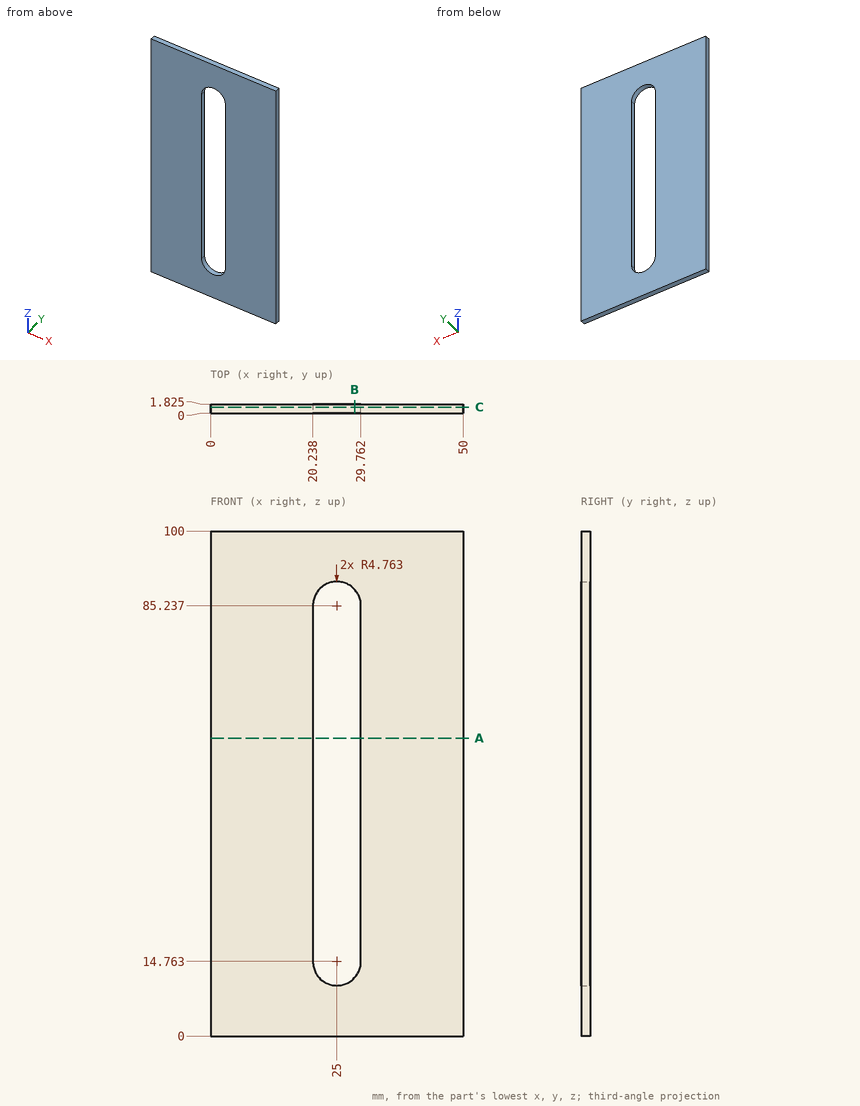
The figure shows three views and two pictorial views of one solid part (mm, origin at its lowest corner). Answer the questions. Round coordinates to 2 decimals unless told otherwise and drop trailing zeros. Write each loop counter-clockwise with the first axis right and the second up, starting at its lowest first coordinate (ties: lowest second). Pieces come first, ordered by that corner, then holes. Notation, with made-up numbers: (34, 48) - (46, 48) arc R9 cw to (46, 55) - close; hole circle Ø10 at (46.5, 42.5). An arc over 180 degrees is marked (long way). Answer in a Markdown table with one row per item. Add a question column.
1. A cutting plane is placed at B-B, the plane x = 28.5. Determine the outline of the cut face in (y, z) (1 decimal).
2. Find the intervals of material crossed by line 1 along X through (y, z) = (1.1, 36); line 2 along X through (y, z) = (0.55, 86.5); line 3 along Z through (x, y) = (28, 0.75) (1 decimal), in increasing order. Write a range as from..to.
3. A cutting plane is placed at A-A, the plane z = 59. Determine the outline of the cut face in (x, y) (1 decimal).
4. A cutting plane is placed at C-C, the plane y = 1.2. Determine the outline of the cut face in (x, z) (1 decimal), and give its area (3 significant figures).
Worked out:
| question | item | result |
|---|---|---|
| 1 | outline | (0, 0) - (1.8, 0) - (1.8, 11.5) - (0, 11.5) - close; (0, 88.5) - (1.8, 88.5) - (1.8, 100) - (0, 100) - close |
| 2 | line 1 | 0..20.24, 29.76..50 |
| 2 | line 2 | 0..20.41, 29.59..50 |
| 2 | line 3 | 0..11.1, 88.9..100 |
| 3 | outline | (0, 0) - (20.2, 0) - (20.2, 1.8) - (0, 1.8) - close; (29.8, 0) - (50, 0) - (50, 1.8) - (29.8, 1.8) - close |
| 4 | outline | (0, 0) - (50, 0) - (50, 100) - (0, 100) - close; hole (20.2, 14.8) arc R4.8 ccw to (29.8, 14.8) - (29.8, 85.2) arc R4.8 ccw to (20.2, 85.2) - close |
| 4 | area | 4,260 mm^2 |
